Model file for the job. Use its own axes, mm. A direction names the side the tool comes from. Round coordinates to 2 decimals unless told otherwise and drop trailing zeros. Order: outer loops, then holes, each group sorted by start corner. A loop starts at its lowest first (then second) coordinate and runs counter-clockwise, first axis right, second up. Notation, with made-up numbers: (1, 53.5) - (48, 53.5) arc R14 ccw to (48, 65.5) - close; hole circle Ø8 at (6, 21). An arc over 180 degrees is marked (long way). Put each result on its own line as item: value. Start each with the question number.
Item 1: Saw through at A-A on x = -140. List the corners of the cut face in (y, z).
Item 2: Saw through at B-B on y = 254. List the corners of the cut face in (x, z).
Item 3: Mould opens along X. For faces 1 (the face through (-28.68, 271.77, -0.22)), 2 (the face through (-172.098, 212.362, -1.502)), 3 (the face through (-101, 242, -25)), 4 (the face through (-34.649, 269.174, -23.574)) say: pulls with the +X half, pulls with the -X half, needs draft (parallel to the pull), parting line crosses it, or undercut.
Item 4: Which spindle directions (+Z, -Z, +X, -X, +Y, -Y) get a long thin tool onto all of the face, cutting with end or side? Do faces 5 (the face through (-34.58, 269.2, 23.5)), 6 (the face through (-167.266, 214.364, 0.28)), 7 (the face through (-99, 241, 40)). Say none if no direction does.
Item 5: Saw through at C-C on z = -32.5. List the corners of the cut face in (x, y).
Item 6: Probe probe 1 along X at (y, z) = (277, 12); probe 2 along Y at (x, z) = (-134, -26.5); probe 3 along Y at (x, z) = (-24.5, -34). List the from-to ranges inside material, lowest first.
Item 7: Pin check, flat tips, straight feed: pin 1 Ø4 at (y, z) = (211.5, -18) entering from +X; pin 2 Ø2 at (y, z) = (258.5, -25.5) entering from -X. Stop position of each tip, or through.
Autodesk Inventor part; units mm, degrees
ref_plane "YZ Plane" through (0, 0, 0) normal (1, 0, 0) x (0, 1, 0)
ref_plane "XZ Plane" through (0, 0, 0) normal (0, 1, 0) x (-1, 0, 0)
ref_plane "XY Plane" through (0, 0, 0) normal (0, 0, 1) x (1, 0, 0)
sketch "Sketch2" plane through (0, 0, 0) normal (0, 0, 1) x (1, 0, 0)
  line L0 (0, 273.8452) -> (193.6378, 193.6378) construction
  line L1 (193.6378, 193.6378) -> (273.8452, 0) construction
  line L2 (273.8452, 0) -> (193.6378, -193.6378) construction
  line L3 (193.6378, -193.6378) -> (0, -273.8452) construction
  line L4 (0, -273.8452) -> (-193.6378, -193.6378) construction
  line L5 (-193.6378, -193.6378) -> (-273.8452, 0) construction
  line L6 (-273.8452, 0) -> (-193.6378, 193.6378) construction
  line L7 (-193.6378, 193.6378) -> (0, 273.8452) construction
  line L8 (-193.6378, 193.6378) -> (0, 273.8452) construction
  line L9 (-459.9272, 770.6562) -> (-219.7185, 870.1539) construction
  line L10 (-96.8189, 233.7415) -> (-339.8229, 820.405) construction
  line L11 (-219.7185, 870.1539) -> (0, 870.1539) construction
  line L12 (0, 870.1539) -> (0, 273.8452) construction
  line L13 (-459.9272, 770.6562) -> (-615.2917, 615.2917) construction
  line L14 (-615.2917, 615.2917) -> (-193.6378, 193.6378) construction
  line L15 (-5, 277.1861) -> (-192.4647, 199.5357) construction
  line L16 (-192.4647, 199.5357) -> (-608.2206, 615.2917) construction
  line L17 (-608.2206, 615.2917) -> (-457.095, 766.4174) construction
  line L18 (-457.095, 766.4174) -> (-218.724, 865.1539) construction
  line L19 (-218.724, 865.1539) -> (-5, 865.1539) construction
  line L20 (-5, 865.1539) -> (-5, 277.1861) construction
  line L21 (-13, 282.5315) -> (-190.5876, 208.9724) construction
  line L22 (-190.5876, 208.9724) -> (-596.9069, 615.2917) construction
  line L23 (-596.9069, 615.2917) -> (-452.5633, 759.6353) construction
  line L24 (-452.5633, 759.6353) -> (-217.1327, 857.1539) construction
  line L25 (-217.1327, 857.1539) -> (-13, 857.1539) construction
  line L26 (-13, 857.1539) -> (-13, 282.5315) construction
  line L27 (-5, 277.1861) -> (-192.4647, 199.5357)
  line L28 (-192.4647, 199.5357) -> (-190.5876, 208.9724)
  line L29 (-190.5876, 208.9724) -> (-13, 282.5315)
  line L30 (-13, 282.5315) -> (-5, 277.1861)
  point P0 (0, 0)
  point P1 (0, 0)
  point P2 (0, 0)
  dimension "d0" = 506
  dimension "d1" = 260
  dimension "d2" = 635
  dimension "d6" = 5
  dimension "d7" = 8
extrude "Extrusion1" add sketch "Sketch2" along normal mid plane 80
sketch "Sketch3" plane through (-13, 282.5315, -40) normal (-0.3827, 0.9239, 0) x (0.9239, 0.3827, 0)
  line L0 (-168.6097, -15) -> (-23.6097, -15)
  line L1 (-23.6097, -15) -> (-23.6097, -65)
  line L2 (-23.6097, -65) -> (-168.6097, -65)
  line L3 (-168.6097, -65) -> (-168.6097, -15)
  circle A0 centre (-13.6097, -40) radius 5
  circle A1 centre (-178.6097, -40) radius 5
  line L4 (0, -80) -> (-192.2194, -80)
  line L5 (-96.1097, -40) -> (-96.1097, -80) construction
  line L6 (5.3454, 0) -> (5.3454, -80) construction
  point P0 (-96.1097, -15)
  point P1 (-168.6097, -40)
  point P2 (-23.6097, -40)
  point P3 (5.3454, -40)
  dimension "d10" = 145
  dimension "d11" = 10
  dimension "d12" = 10
  dimension "d13" = 50
extrude "Extrusion2" cut sketch "Sketch3" against normal up to surface (8 mm away)
fillet "Fillet1" radius 5 4 edges at (-167.2443, 214.3119, -25) (-33.2818, 269.801, -25) (-33.2818, 269.801, 25) (-167.2443, 214.3119, 25)
equation "\"d0\" = Барабан_габарит_по_кассетам"
equation "\"d1\" = Кассета_длина_грани"
equation "\"d2\" = Кассета_высота"
equation "\"d10\" = Длина_окна_барабан"
equation "\"d11\" = Диам_шпильки_под_кассету"
equation "\"d13\" = Ширина_окна_барабан"
properties part number "ДМС 204 Нижний лист"
Results found:
1. outline: (221.27, -40) - (229.93, -40) - (229.93, -25) - (221.27, -25) - close; (221.27, 25) - (229.93, 25) - (229.93, 40) - (221.27, 40) - close
2. outline: (-81.88, -40) - (-60.98, -40) - (-60.98, -25) - (-81.88, -25) - close; (-81.88, 25) - (-60.98, 25) - (-60.98, 40) - (-81.88, 40) - close
3. face 1: undercut
3. face 2: undercut
3. face 3: needs draft
3. face 4: pulls with the -X half
4. face 5: -X, -Y
4. face 6: +X, +Y
4. face 7: +Z, +X, -X, +Y, -Y
5. outline: (-192.46, 199.54) - (-5, 277.19) - (-13, 282.53) - (-190.59, 208.97) - close
6. probe 1: x = -26.35 to -5.45
6. probe 2: y = 223.75 to 232.41
6. probe 3: y = 269.11 to 277.77
7. pin 1: stops at x = -165.71
7. pin 2: stops at x = -73.43
